from build123d import *

# Parameters (mm, degrees)
EXTRUDE_1_DEPTH     = 1.2
SKETCH_2_W          = 181
SKETCH_2_H          = 66.6
EXTRUDE_2_DEPTH     = 6
SKETCH_3_W          = 175.952774737
SKETCH_3_H          = 62.140674221
EXTRUDE_3_DEPTH     = 0.2
SKETCH_4_W          = 181
SKETCH_4_H          = 66.6
EXTRUDE_4_DEPTH     = 1.6
SKETCH_5_W          = 161.4
SKETCH_5_H          = 61.02
CUT_EXTRUDE_1_DEPTH = 0.01
SKETCH_7_W          = 4.5
SKETCH_7_H          = 25
EXTRUDE_5_DEPTH     = 2


with BuildPart() as part:
    # Эскиз1 (on Right Plane) → Бобышка-Вытянуть1 (new body)
    with BuildSketch(Plane(origin=(0, 0, 0), x_dir=(0, 0, -1), z_dir=(1, 0, 0))):
        with BuildLine():
            Line((91.6, -38.4), (-91.6, -38.4))
            ThreePointArc((-91.6, -38.4), (-93.721320344, -37.521320344), (-94.6, -35.4))
            Line((-94.6, -35.4), (-94.6, 35.4))
            ThreePointArc((-94.6, 35.4), (-93.721320344, 37.521320344), (-91.6, 38.4))
            Line((-91.6, 38.4), (91.6, 38.4))
            ThreePointArc((91.6, 38.4), (93.721320344, 37.521320344), (94.6, 35.4))
            Line((94.6, 35.4), (94.6, -35.4))
            ThreePointArc((94.6, -35.4), (93.721320344, -37.521320344), (91.6, -38.4))
        make_face()
    extrude(amount=EXTRUDE_1_DEPTH)

    # Эскиз2 → Бобышка-Вытянуть2 (add)
    with BuildSketch(Plane(origin=(1.2, 0, 0), x_dir=(0, 0, -1), z_dir=(1, 0, 0))):
        Rectangle(SKETCH_2_W, SKETCH_2_H)
    extrude(amount=EXTRUDE_2_DEPTH)

    # Эскиз3 → Бобышка-Вытянуть3 (add)
    with BuildSketch(Plane(origin=(7.2, 0, 0), x_dir=(0, 0, -1), z_dir=(1, 0, 0))):
        with Locations((0.437545425, -0.270444937)):
            Rectangle(SKETCH_3_W, SKETCH_3_H)
    extrude(amount=EXTRUDE_3_DEPTH)

    # Эскиз4 → Бобышка-Вытянуть4 (add)
    with BuildSketch(Plane(origin=(7.4, 0, 0), x_dir=(0, 0, -1), z_dir=(1, 0, 0))):
        Rectangle(SKETCH_4_W, SKETCH_4_H)
    extrude(amount=EXTRUDE_4_DEPTH)

    # Эскиз5 → Вырез-Вытянуть1 (cut)
    with BuildSketch(Plane.ZY):
        Rectangle(SKETCH_5_W, SKETCH_5_H)
    extrude(amount=-CUT_EXTRUDE_1_DEPTH, mode=Mode.SUBTRACT)

    # Эскиз7 → Бобышка-Вытянуть5 (add)
    with BuildSketch(Plane(origin=(9, 0, 0), x_dir=(0, 0, -1), z_dir=(1, 0, 0))):
        with Locations((53.75, 0)):
            Rectangle(SKETCH_7_W, SKETCH_7_H)
    extrude(amount=EXTRUDE_5_DEPTH)


solid = part.part
Read the model definition and answer for the solid it produces. Units are mm, in the model's axes. A direction names the side the tool comes from. Coordinates: 2 decimals unless noted, no trailing zeros. Put each result on its own line as item: value. Start each with the question number.
Item 1: The mould has two halves that part along X. Classify faces 1 (the face through (7.4, -32, 27)), 2 (the face through (0.01, 0, -1)), 3 (the face through (4, 0, -90.5)): +X half, -X half, draft (parallel to the pull), parting line (faces both ways), or undercut.
Item 2: Given pin 1 Ø2 at (y, z) = (-25.5, 9) entering from +X; pin 2 Ø1 at (y, z) = (10.5, 52) entering from -X; pin 3 Ø1.8 at (x, z) = (5, -26) entering from +Y, each flat-ended and moving along its own axis, determine where each tip first touches the part or whether it passes through.
Item 3: For faces 4 (the face through (4, -33.3, 1)), 5 (the face through (11, 0, -54)), 6 (the face through (4, 33.3, 1)), 7 (the face through (4, 0, 90.5)), determine the directions among +Z, -Z, +X, -X, +Y, -Y from which every point of the face is accessible in a straight line to the end or side of a thin tool.
Item 4: Consider probe 1 along X at (y, z) = (-2.5, -43.5); probe 2 along Y at (x, z) = (1.75, 62); probe 3 along Z at (x, y) = (6.75, -9.5). Determine where each line is inside the solid, lowest interval first. Write a range as [from, to].
Computed:
1. face 1: undercut
1. face 2: -X half
1. face 3: draft
2. pin 1: stops at x = 9
2. pin 2: stops at x = 0.01
2. pin 3: stops at y = 33.3
3. face 4: +Z, -Z, +X, -Y
3. face 5: +Z, -Z, +X, +Y, -Y
3. face 6: +Z, -Z, +X, +Y
3. face 7: +Z, +X, +Y, -Y
4. probe 1: x = [0.01, 9]
4. probe 2: y = [-33.3, 33.3]
4. probe 3: z = [-90.5, 90.5]
